The model under review builds one solid part; all positions refer to its coordinate system, in mm. A direction names the side the tool comes from. Give positions to 0.01 mm unless a question says otherwise; leave off trailing zeros. Order: outer loops, then holes, each group sorted by start corner. A loop starts at its lowest first (then second) coordinate and runs counter-clockwise, first axis right, second up.
```python
from build123d import *

# Parameters (mm, degrees)
F0_W      = 2000
F0_H      = 1000
F1_DEPTH  = 25
F2_W      = 100
F2_H      = 100
F3_DEPTH  = 700
F5_W      = 100
F5_H      = 100
F6_DEPTH  = 673
F7_D      = 50
F8_R      = 25
F9_DEPTH  = 25
F9_FACE_R = 25
F10_DEPTH = 975.001
F11_R     = 30


with BuildPart() as f1:
    # F0 (on Front) → F1 (new body)
    with BuildSketch(Plane.XZ):
        with Locations((1.290835, 11.492619)):
            Rectangle(F0_W, F0_H)
    extrude(amount=F1_DEPTH)

    # F2 (on Front) → F3 (join)
    with BuildSketch(Plane.XZ):
        with Locations((-898.709165, 411.492619)):
            Rectangle(F2_W, F2_H)
    extrude(amount=F3_DEPTH)

    # F5 (on face) → F6 (join)
    with BuildSketch(Plane.XZ.offset(25)):
        with Locations((-898.709165, -388.507381)):
            Rectangle(F5_W, F5_H)
        with Locations((901.290835, -388.507381)):
            Rectangle(F5_W, F5_H)
        with Locations((901.290835, 411.492619)):
            Rectangle(F5_W, F5_H)
    extrude(amount=F6_DEPTH)

    # F7 (through all)
    with Locations(Plane.XY.offset(461.492619)):
        with Locations((-898.709165, -500)):
            Hole(F7_D / 2)

    # F8 (on face) → F9 (join)
    with BuildSketch(Plane.XY.offset(461.492619)):
        with Locations((-898.709165, -300)):
            Circle(F8_R)
        with Locations((-898.709165, -100)):
            Circle(F8_R)
        with Locations((-898.709165, -500)):
            Circle(F8_R)
        with Locations((901.290835, -498)):
            Circle(F8_R)
        with Locations((901.290835, -298)):
            Circle(F8_R)
        with Locations((901.290835, -98)):
            Circle(F8_R)
    extrude(amount=F9_DEPTH)

    # F9_face (on face) → F10 (cut, through all)
    with BuildSketch(Plane(origin=(-898.709165, -300, 486.492619), x_dir=(1, 0, 0), z_dir=(0, 0, 1))):
        Circle(F9_FACE_R)
        with Locations((0, 200)):
            Circle(F9_FACE_R)
        with Locations((0, -200)):
            Circle(F9_FACE_R)
        with Locations((1800, 202)):
            Circle(F9_FACE_R)
        with Locations((1800, 2)):
            Circle(F9_FACE_R)
        with Locations((1800, -198)):
            Circle(F9_FACE_R)
    extrude(amount=-F10_DEPTH, mode=Mode.SUBTRACT)

    # F11
    f11_edges = [f1.edges().sort_by_distance(p)[0] for p in [
        (-998.709165, -12.5, 511.492619),
        (-998.709165, -12.5, -488.507381),
        (1001.290835, -12.5, -488.507381),
        (1001.290835, -12.5, 511.492619),
    ]]
    fillet(f11_edges, radius=F11_R)


solid = f1.part
```
Item 1: Draft analysis for pull direction X (two halves, no side actions). For faces 1 (the flat face through (951.291, -357, 411)), 2 (the cylindrical face through (-901.964, -275.213, -387.807)), 3 (the flat face through (901, -698, 412)), 4 (the cylindrical face through (898.036, -473.213, -387.807)), state which applies: released by +X, released by -X, zero draft, split by the parting line, or undercut.
Values found:
face 1: released by +X
face 2: undercut
face 3: zero draft
face 4: undercut
Item 2: Take a section at A-A (y = -592.5). Give the boundary of the cut face in (x, z), and give its area (3 significant figures).
Values found:
outline: (-948.71, -438.51) - (-848.71, -438.51) - (-848.71, -338.51) - (-948.71, -338.51) - close; (-948.71, 361.49) - (-848.71, 361.49) - (-848.71, 461.49) - (-948.71, 461.49) - close; (851.29, -438.51) - (951.29, -438.51) - (951.29, -338.51) - (851.29, -338.51) - close; (851.29, 361.49) - (951.29, 361.49) - (951.29, 461.49) - (851.29, 461.49) - close
area: 40,000 mm2
Item 3: Take a section at C-C (x = -60.5). Give the boundary of the cut face in (y, z).
Values found:
outline: (-25, -488.51) - (0, -488.51) - (0, 511.49) - (-25, 511.49) - close
Item 4: For faces 5 (the flat face through (-899, -357, -438.507)), 6 (the flat face through (-899, -358, 361.493)), 7 (the flat face through (-948.709, -358, 411)), 8 (the flat face through (851.291, -357, 411)), list the 3-axis set-ups (+Z, -Z, +X, -X, +Y, -Y) from which the entire face can be reached by the end or side of a thin tool; tool diameter is ignored.
Values found:
face 5: -Z, +X, -X, -Y
face 6: +X, -X, -Y
face 7: +Z, -Z, -X, -Y
face 8: +Z, -Z, -Y
Item 5: Clearance check with flat-ended pins moving along their axes: pin 1 Ø8 at (x, z) = (-66, 20) entering from -Y; pin 2 Ø2 at (x, z) = (-499.5, 304.5) entering from +Y. State where each tip first meets the part, or that it passes through.
Values found:
pin 1: stops at y = -25
pin 2: stops at y = 0
Item 6: Take a section at D-D (z = 145). Give the boundary of the cut face in (x, y).
Values found:
outline: (-998.71, -25) - (1001.29, -25) - (1001.29, 0) - (-998.71, 0) - close
Item 7: For line 1 (Y direction, x = -212, z = 54); line 2 (Y direction, x = -905, z = -380), list the stretches that pass through material, from the lowest coordinate up.
Values found:
line 1: y = -25 to 0
line 2: y = -698 to -524.2, -475.8 to -324.2, -275.8 to -124.2, -75.8 to 0
Item 8: Take a section at B-B (z = 416). Give the boundary of the cut face in (x, y), and give its area (3 significant figures).
Values found:
outline: (-998.71, -25) - (-948.71, -25) - (-948.71, -700) - (-848.71, -700) - (-848.71, -25) - (851.29, -25) - (851.29, -698) - (951.29, -698) - (951.29, -25) - (1001.29, -25) - (1001.29, 0) - (-998.71, 0) - close; hole circle Ø50 at (-898.71, -500); hole circle Ø50 at (-898.71, -300); hole circle Ø50 at (-898.71, -100); hole circle Ø50 at (901.29, -498); hole circle Ø50 at (901.29, -298); hole circle Ø50 at (901.29, -98)
area: 173,000 mm2
